Autodesk Inventor part; units mm, degrees
ref_plane "YZ Plane" through (0, 0, 0) normal (1, 0, 0) x (0, 1, 0)
ref_plane "XZ Plane" through (0, 0, 0) normal (0, 1, 0) x (-1, 0, 0)
ref_plane "XY Plane" through (0, 0, 0) normal (0, 0, 1) x (1, 0, 0)
sketch "Sketch1" plane through (0, 0, 0) normal (0, 1, 0) x (-1, 0, 0)
  circle A0 centre (0, 0) radius 1.5
  dimension "d0" = 3
extrude "Extrusion1" add sketch "Sketch1" along normal blind 9.7
sketch "Sketch2" plane through (0, 9.7, 0) normal (0, 1, 0) x (1, 0, 0)
  circle A0 centre (0, 0) radius 2.75
  dimension "d3" = 5.5
extrude "Extrusion2" add sketch "Sketch2" along normal blind 2.2
sketch "Sketch3" plane through (0, 11.9, 0) normal (0, 1, 0) x (1, 0, 0)
  line L0 (0.5, -4.7072) -> (-0.5, -4.7072)
  line L1 (-0.5, -4.7072) -> (-0.5, 4.7072)
  line L2 (-0.5, 4.7072) -> (0.5, 4.7072)
  line L3 (0.5, 4.7072) -> (0.5, -4.7072)
  line L4 (0.5, -4.7072) -> (-0.5, 4.7072) construction
  line L5 (-0.5, -4.7072) -> (0.5, 4.7072) construction
  point P0 (0, 0)
  dimension "d6" = 1
extrude "Extrusion3" cut sketch "Sketch3" against normal blind 1
properties part number "screw12x3mm" material "Stainless Steel"
Read the model definition and answer for the solid it produces. Units are mm, in the model's axes. A direction names the side the tool comes from. Give positions to 0.01 mm unless a question says otherwise; leave off trailing zeros. Loops run counter-clockwise (first coordinate to the right, second up) from the corner with the lowest first, then second, coordinate; pieces in that order, holes last. Notation, with made-up numbers: (9.5, 13.25) -> (17.5, 13.25) arc R16 cw to (17.5, 38.25) -> close; hole circle Ø2 at (4.25, 57.5). An arc over 180 degrees is marked (long way). Use a Markdown table: item, result.
Q1. Find the intervals of material crossed by line 1 along Y through (x, z) = (0.75, -1.7); line 2 along X through (y, z) = (11.25, 0.65); line 3 along Y through (x, z) = (0, 1.6), in increasing order.
Solved:
| item | result |
|---|---|
| line 1 | y = 9.7 to 11.9 |
| line 2 | x = -2.67 to -0.5, 0.5 to 2.67 |
| line 3 | y = 9.7 to 10.9 |
Q2. Each of these flat-tipped pins is pushed along its axis until it touches: pin 1 (0.5 mm diameter, centred on x = 0, z = -0.5, fed in from +Y); pin 2 (1.1 mm diameter, centred on y = 11.5, z = -1, fed in from -X); pin 3 (2 mm diameter, centred on x = -1, z = 1.5, fed in from -Y); pin 4 (0.8 mm diameter, centred on y = 11, z = 0.5, fed in from +X). Where does it stop, or does it pass through?
Solved:
| item | result |
|---|---|
| pin 1 | stops at y = 10.9 |
| pin 2 | stops at x = -2.71 |
| pin 3 | stops at y = 0 |
| pin 4 | stops at x = 2.75 |
Q3. Section A-A, the plane x = 0 is taken. Determine the outline of the cut face in (y, z), then the cut area to 3 significant figures.
Solved:
| item | result |
|---|---|
| outline | (0, -1.5) -> (9.7, -1.5) -> (9.7, -2.75) -> (10.9, -2.75) -> (10.9, 2.75) -> (9.7, 2.75) -> (9.7, 1.5) -> (0, 1.5) -> close |
| area | 35.7 mm^2 |
Q4. A tool of negligible diameter and unlimited length cuts with its end or side. For faces 1 (the face through (-0.5, 11.4, 0)), 2 (the face through (1.5, 4.78, -0.07)), 3 (the face through (0, 0, 0)), from which of +Z, -Z, +X, -X, +Y, -Y can it reach the whole face along a straight path? Write none if from no direction.
Solved:
| item | result |
|---|---|
| face 1 | +Z, -Z, +Y |
| face 2 | -Y |
| face 3 | +Z, -Z, +X, -X, -Y |
Q5. Section B-B, the plane z = 0 is taken. Determine the outline of the cut face in (x, y).
Solved:
| item | result |
|---|---|
| outline | (-2.75, 9.7) -> (-1.5, 9.7) -> (-1.5, 0) -> (1.5, 0) -> (1.5, 9.7) -> (2.75, 9.7) -> (2.75, 11.9) -> (0.5, 11.9) -> (0.5, 10.9) -> (-0.5, 10.9) -> (-0.5, 11.9) -> (-2.75, 11.9) -> close |
Q6. Section C-C, the plane y = 10.75 is taken. Determine the outline of the cut face in (x, z), then the cut area to 3 significant figures.
Solved:
| item | result |
|---|---|
| outline | circle Ø5.5 at (0, 0) |
| area | 23.8 mm^2 |
Q7. Section D-D, the plane x = -0.9 is taken. Determine the outline of the cut face in (y, z), then the cut area to 3 significant figures.
Solved:
| item | result |
|---|---|
| outline | (0, -1.2) -> (9.7, -1.2) -> (9.7, -2.6) -> (11.9, -2.6) -> (11.9, 2.6) -> (9.7, 2.6) -> (9.7, 1.2) -> (0, 1.2) -> close |
| area | 34.7 mm^2 |
Q8. Determine the mould class of faces 4 (the face through (0.5, 11.4, 0)), 5 (the face through (1.27, 10.78, -2.44)), 6 (the face through (-1, 11.9, 0)) for opening direction X: pulls with the +X half, pulls with the -X half, needs draft (parallel to the pull), parting line crosses it, or undercut.
Solved:
| item | result |
|---|---|
| face 4 | undercut |
| face 5 | parting line crosses it |
| face 6 | needs draft |
